Here's how the part is built. I have some questions about the finished solid (model axes, mm). Round coordinates to 2 decimals unless told otherwise and drop trailing zeros. Write each loop counter-clockwise with the first axis right and the second up, starting at its lowest first coordinate (ties: lowest second). Pieces come first, ordered by that corner, then holes. Notation, with made-up numbers: (20, 31.25) - (79, 31.25) arc R21 ccw to (79, 37.25) - close; hole circle Ø7 at (80, -23). An arc over 180 degrees is marked (long way). Use one line per item in the form item = value. Start each with the question number.
1. I want a section at B-B, the plane z = 368.5. List the corners of the cut face in (x, y) for me, plus the area to 3 significant figures.
2. If I drill on line 1 along Y through (x, z) = (0, 917.5); line 2 along Y through (x, z) = (1.5, 375), over which ranges is the centre line in solid material (lowest first)?
3. Will these pins go through, and if not, where does the flat tip stop? pin 1 (10 mm diameter, centred on y = 8, z = 412.5, fed in from +X); pin 2 (1.5 mm diameter, centred on x = -8, z = 1266, fed in from +Y); pin 3 (5 mm diameter, centred on x = -10.5, z = 169.5, fed in from -Y).
4. We'd pull the mould along X, two halves only. Please class faces 1 (the cylindrical face through (-3.62, 16.303, 726.288)), 2 (the cylindrical face through (12.707, -4.002, 726.288)), 3 (the flat face through (-1, -14, 1473.2)): +X half, -X half, draft (parallel to the pull), parting line (faces both ways), or undercut.
5. I want a section at A-A, the plane y = 0. List the corners of the cut face in (x, z) for me.
Autodesk Inventor part; units mm, degrees
ref_plane "Start plane" through (0, 0, 0) normal (0, 0, 1) x (1, 0, 0)
ref_plane "End plane" through (0, 0, 1473.2) normal (0, 0, 1) x (1, 0, 0)
ref_plane "Work Plane4" through (0, 0, 1193.8) normal (-1, 0, 0) x (0, 0, 1)
ref_plane "Start plane" through (0, 0, 0) normal (0, 0, 1) x (1, 0, 0)
ref_plane "End plane" through (0, 0, 1473.2) normal (0, 0, 1) x (1, 0, 0)
sketch "Sketch" plane through (0, 0, 0) normal (0, 0, 1) x (1, 0, 0)
  circle A0 centre (0, 0) radius 13.3223
  circle A1 centre (0, 0) radius 16.7005
  dimension "d0" = 33.401
  dimension "d1" = 3.3782
extrude "Body" add sketch "Sketch" along normal up to surface (1473.2 mm away) from surface at 0
sketch "Sketch3" plane through (0, 0, 0) normal (0, 0, 1) x (1, 0, 0)
  line L0 (0, 0) -> (10, 0)
ref_plane "Work Plane3" through (0, 0, 0) normal (0, -1, 0) x (1, 0, 0)
sketch "Sketch4" plane through (0, 0, 0) normal (0, -1, 0) x (1, 0, 0)
  line L0 (-2, 0) -> (12, 0)
  line L1 (-2, 1473.2) -> (12, 1473.2)
  dimension "d7" = 1473.2
ref_plane "Work Plane4" through (0, 0, 1193.8) normal (-1, 0, 0) x (0, 0, 1)
ref_plane "Work Plane5" through (-2143.252, 0, 1193.8) normal (-1, 0, 0) x (0, 0, 1)
ref_plane "Work Plane6" through (-1071.626, 0, 1193.8) normal (-1, 0, 0) x (0, 0, 1)
sketch "Sketch5" plane through (-1071.626, 0, 1193.8) normal (-1, 0, 0) x (0, 0, 1)
  circle A0 centre (0, 0) radius 16.7005
  circle A1 centre (0, 0) radius 13.3223
extrude "Extrusion2" cut sketch "Sketch5" along normal up to surface (2143.252 mm away) from surface at -1071.626 contours A0 | A1
equation "\"d0\" = G_H"
equation "\"d1\" = G_T"
equation "\"d2\" = G_L"
equation "\"G_H\" = 33.401"
equation "\"G_T\" = 3.3782"
equation "\"G_L\" = d7"
equation "\"G_OFFSET_START\" = 0"
equation "\"G_OFFSET_END\" = 0"
equation "\"d5\" = G_OFFSET_END + B_L"
equation "\"B_L\" = 1473.2"
properties part number "ANSI - 1 x 0.133 - 58" material "Aluminum 6061"
Model answer:
q1.outline = circle Ø33.4 at (0, 0); hole circle Ø26.64 at (0, 0)
q1.area = 319 mm2
q2.line_1 = -16.7 to -13.32, 13.32 to 16.7
q2.line_2 = -16.63 to -13.24, 13.24 to 16.63
q3.pin_1 = 16.43
q3.pin_2 = 15.04
q3.pin_3 = -14.66
q4.face_1 = parting line
q4.face_2 = undercut
q4.face_3 = draft
q5.outline = (-16.7, 0) - (-13.32, 0) - (-13.32, 1177.1) - (-16.7, 1177.1) - close; (-16.7, 1210.5) - (-13.32, 1210.5) - (-13.32, 1473.2) - (-16.7, 1473.2) - close; (13.32, 0) - (16.7, 0) - (16.7, 1473.2) - (13.32, 1473.2) - close
